Drawing for the job (mm, zero at the part's lowest x, y, z). A direction names the side the tool comes from. Coordinates: 2 decimals unless noted, no trailing zeros. Write each loop counter-clockwise with the first axis right and the second up, starting at its lowest first coordinate (ties: lowest second). Pieces come first, ordered by that corner, then holes. Notation, with made-up numbers: (-25.5, -10) - (9.5, -10) arc R19 ccw to (9.5, -6) - close; hole circle Ø2 at (-40, 18.5). An arc over 180 degrees is marked (long way). Write each question's results on one line, items separated by ' | '.
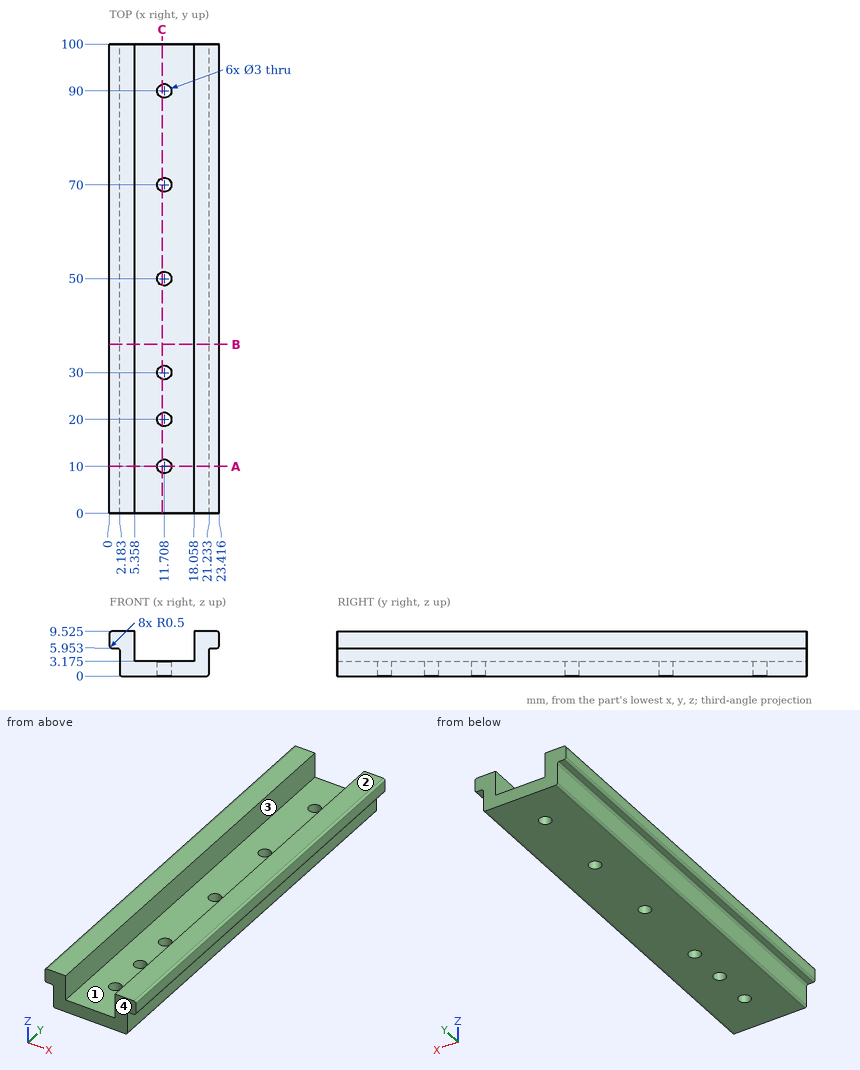
(1) Flat gauge pins, fed straight in: P1, Ø2.5, axis at x = 11.71, y = 20, coming from the +Z side; P2, Ø4, axis at y = 30, z = 2, coming from the +X side; P3, Ø10, axis at x = 12.5, y = 70, coming from the +Z side (3 decimals); P4, Ø1.5, axis at y = 35.5, z = 3, coming from the -X side. Where does each tip first touch, or does it go through?
Return value:
P1: passes through | P2: stops at x = 21.23 | P3: stops at z = 3.175 | P4: stops at x = 2.18
(2) Two-plate mould, pull along X, no slides. Class the marked faces 3 and 4: released by +X, released by -X, zero draft, split by the parting line, or undercut.
Return value:
face 3: undercut | face 4: zero draft
(3) Saw through at A-A on y = 10. Write the cut outline in (x, z) (1 decimal).
Return value:
outline: (0, 6.5) arc R0.5 ccw to (0.5, 6) - (1.7, 6) arc R0.5 cw to (2.2, 5.5) - (2.2, 0.5) arc R0.5 ccw to (2.7, 0) - (10.2, 0) - (10.2, 3.2) - (5.4, 3.2) - (5.4, 9.5) - (0.5, 9.5) arc R0.5 ccw to (0, 9) - close; (13.2, 0) - (20.7, 0) arc R0.5 ccw to (21.2, 0.5) - (21.2, 5.5) arc R0.5 cw to (21.7, 6) - (22.9, 6) arc R0.5 ccw to (23.4, 6.5) - (23.4, 9) arc R0.5 ccw to (22.9, 9.5) - (18.1, 9.5) - (18.1, 3.2) - (13.2, 3.2) - close
(4) Wall check: line 1 (X direction, y = 10, z = 6.5) (1 decimal); line 2 (X direction, y = 27.5, z = 4); line 3 (Z direction, x = 17, y = 18) (1 decimal). Give the ranges that are in metal, low to high. Write a range as from..to.
Return value:
line 1: x = 0..5.4, 18.1..23.4 | line 2: x = 2.18..5.36, 18.06..21.23 | line 3: z = 0..3.2
(5) Saw through at B-B on y = 36. Write the cut outline in (x, z) (1 decimal).
Return value:
outline: (0, 6.5) arc R0.5 ccw to (0.5, 6) - (1.7, 6) arc R0.5 cw to (2.2, 5.5) - (2.2, 0.5) arc R0.5 ccw to (2.7, 0) - (20.7, 0) arc R0.5 ccw to (21.2, 0.5) - (21.2, 5.5) arc R0.5 cw to (21.7, 6) - (22.9, 6) arc R0.5 ccw to (23.4, 6.5) - (23.4, 9) arc R0.5 ccw to (22.9, 9.5) - (18.1, 9.5) - (18.1, 3.2) - (5.4, 3.2) - (5.4, 9.5) - (0.5, 9.5) arc R0.5 ccw to (0, 9) - close
(6) 3-axis set-ups, long thin cutter, end or side, ignore diameter. For the marked faces 1 and 2: which of +Z, -Z, +X, -X, +Y, -Y reach the whole face in a straight line?
Return value:
face 1: +Z, +Y, -Y | face 2: +Z, +X, -X, +Y, -Y
(7) Saw through at C-C on x = 11.25. Write the cut outline in (y, z) (1 decimal).
Return value:
outline: (0, 0) - (8.6, 0) - (8.6, 3.2) - (0, 3.2) - close; (11.4, 0) - (18.6, 0) - (18.6, 3.2) - (11.4, 3.2) - close; (21.4, 0) - (28.6, 0) - (28.6, 3.2) - (21.4, 3.2) - close; (31.4, 0) - (48.6, 0) - (48.6, 3.2) - (31.4, 3.2) - close; (51.4, 0) - (68.6, 0) - (68.6, 3.2) - (51.4, 3.2) - close; (71.4, 0) - (88.6, 0) - (88.6, 3.2) - (71.4, 3.2) - close; (91.4, 0) - (100, 0) - (100, 3.2) - (91.4, 3.2) - close
